Autodesk Inventor part; units mm, degrees
ref_plane "Work Plane1" through (29, 0, 0) normal (0, -1, 0) x (1, 0, 0)
ref_plane "YZ Plane" through (0, 0, 0) normal (1, 0, 0) x (0, 1, 0)
ref_plane "XZ Plane" through (0, 0, 0) normal (0, 1, 0) x (-1, 0, 0)
sketch "Sketch1" plane through (0, 0, 0) normal (0, 0, 1) x (1, 0, 0)
  line L0 (-1, 0) -> (20, 0)
  line L1 (20, 0) -> (20, 2)
  line L2 (20, 2) -> (6, 2)
  line L3 (6, 2) -> (5.5705, 2)
  line L4 (5.5705, 2) -> (0, 2)
  line L5 (0, 2) -> (0, 3.5)
  line L6 (0, 3.5) -> (-4, 3.5)
  line L7 (-4, 3.5) -> (-4, 1.7321)
  line L8 (-4, 1.7321) -> (-2, 1.7321)
  line L9 (-2, 1.7321) -> (-1, 0)
  line L10 (-8.8, 0) -> (24.8, 0)
  line L11 (0, -0.7) -> (0, 4.2)
  line L12 (6, 2) -> (0, 2) construction
  dimension "d1" = 14
  dimension "d2" = 0.4295
  dimension "d3" = 4
  dimension "d4" = 2
  dimension "d5" = 60
  dimension "d6" = 4
  dimension "d7" = 4
  dimension "d8" = 3.4641
  dimension "d9" = 7
  dimension "d26" = 20
revolve "Body" add sketch "Sketch1" angle 360 about axis through (-1, 0, 0) along (1, 0, 0)
sketch "Sketch2" plane through (-4, 0, 0) normal (-1, 0, 0) x (0, 0, 1)
  circle A0 centre (0, 0) radius 1.7321
  line L0 (0, -4.9) -> (0, 4.9)
  line L1 (-4.9, 0) -> (4.9, 0)
  line L2 (1.7321, 0) -> (0.866, -1.5)
  line L3 (0.866, -1.5) -> (-0.866, -1.5)
  line L4 (-0.866, -1.5) -> (-1.7321, 0)
  line L5 (-1.7321, 0) -> (-0.866, 1.5)
  line L6 (-0.866, 1.5) -> (0.866, 1.5)
  line L7 (0.866, 1.5) -> (1.7321, 0)
extrude "Slot" add sketch "Sketch2" against normal up to next contours L7 A0 | A0 L2 | L6 L0 A0 | A0 L0 L3 | L0 L6 A0 | A0 L3 L0 | L4 A0 | A0 L5
fillet "Fillet1" radius 0.4 1 edges at (-4, -3.5, 0)
thread "Thread"
chamfer "Chamfer1" distance 0.4294 distance2 0.4294 1 edges at (20, -2, 0) measured on face at (20, 0.527, -0.2661)
ref_plane "Work Plane1" through (29, 0, 0) normal (0, -1, 0) x (1, 0, 0)
fillet "Fillet2" radius 0.1 1 edges at (0, -2, 0)
equation "\"d1\" = GEL"
equation "\"d3\" = KOH"
equation "\"d4\" = INTI"
equation "\"d6\" = GD"
equation "\"d7\" = BDM"
equation "\"d8\" = 1.1547 * SW"
equation "\"d9\" = KOD"
equation "\"d26\" = NLG"
equation "\"d30\" = R"
equation "\"d17\" = RR"
equation "\"d13\" = GEL"
equation "\"d15\" = -0.5 * SPD + 0.5 * GD"
equation "\"d16\" = GUL"
equation "\"GD\" = NND"
equation "\"NLG\" = 20"
equation "\"GEL\" = 14"
equation "\"KOD\" = 7"
equation "\"KOH\" = NND"
equation "\"INTI\" = 2"
equation "\"GAL\" = 0.61345 * PTC"
equation "\"GUL\" = 0.61345 * PTC"
equation "\"BDM\" = NND"
equation "\"SW\" = 3"
equation "\"RR\" = 0.1 * NND"
equation "\"SPD\" = NND - 1.2269 * PTC"
equation "\"R\" = 0.1"
equation "\"PHH\" = 0.13"
equation "\"GD1\" = THREADDIA - 1.2269 * PTC"
equation "\"THREADDIA\" = 4"
equation "\"FAWI\" = 45deg"
equation "\"PTC\" = 0.7"
equation "\"KOH1\" = 3.6"
equation "\"NND\" = 4"
equation "\"TOA\" = 30deg"
equation "\"E0\" = 1.155 * SW"
properties part number "AS 1420 - 1973 - M4 x 20" material "Steel, Mild"
Geometry check sheet. Reference: the model listing, model coordinates, mm. A direction names the side the tool comes from. Give positions to 0.01 mm unless a question says otherwise; leave off trailing zeros. Order: outer loops, then holes, each group sorted by start corner. A loop starts at its lowest first (then second) coordinate and runs counter-clockwise, first axis right, second up. Notation, with made-up numbers: (-31, 68.25) - (25, 68.25) arc R29 ccw to (25, 89.25) - close; hole circle Ø7 at (19, 6). An arc over 180 degrees is marked (long way). Write item = value, one per line. Start each with the question number.
1) Access from +Z, -Z, +X, -X, +Y, -Y to the whole of each face (thin tool, end or side, straight path). Record for faces 1 (the flat face through (-2.948, -0.74, 1.305)), 2 (the cylindrical face through (10, 0, 2)), 3 (the flat face through (-4, -1.3, 1.3)).
2) Draft check along Y on faces 4 (the flat face through (20, 0, 0)), 5 (the flat face through (-2.948, 0.74, -1.305)), 6 (the cylindrical face through (-1.825, 3.233, 1.341)). Enter one of: released by +Y, released by -Y, zero draft, split by the parting line, or undercut.
3) Gauge pin test, flat ends, axial feed: pin 1 Ø1 at (x, z) = (13.5, 0.5) entering from -Y; pin 2 Ø0.9 at (x, z) = (-2.5, 0.5) entering from -Y. Record the tip position at first contact, or that the pin passes through.
4) Scan lines: L1, parallel to Z at x = 10.75, y = -1; L2, parallel to X at y = 3, z = 0; L3, parallel to Z at x = 18, y = 0. Record each from-to range of solid material in increasing order.
5) Section check A-A (x = 6). Enter the section's corners in (y, z).
Geometry check:
q1.face_1 = -X
q1.face_2 = +X
q1.face_3 = +Z, -Z, -X, +Y, -Y
q2.face_4 = zero draft
q2.face_5 = undercut
q2.face_6 = split by the parting line
q3.pin_1 = -2
q3.pin_2 = -3.5
q4.L1 = -1.73 to 1.73
q4.L2 = -4 to 0
q4.L3 = -2 to 2
q5.outline = circle Ø4 at (0, 0)
